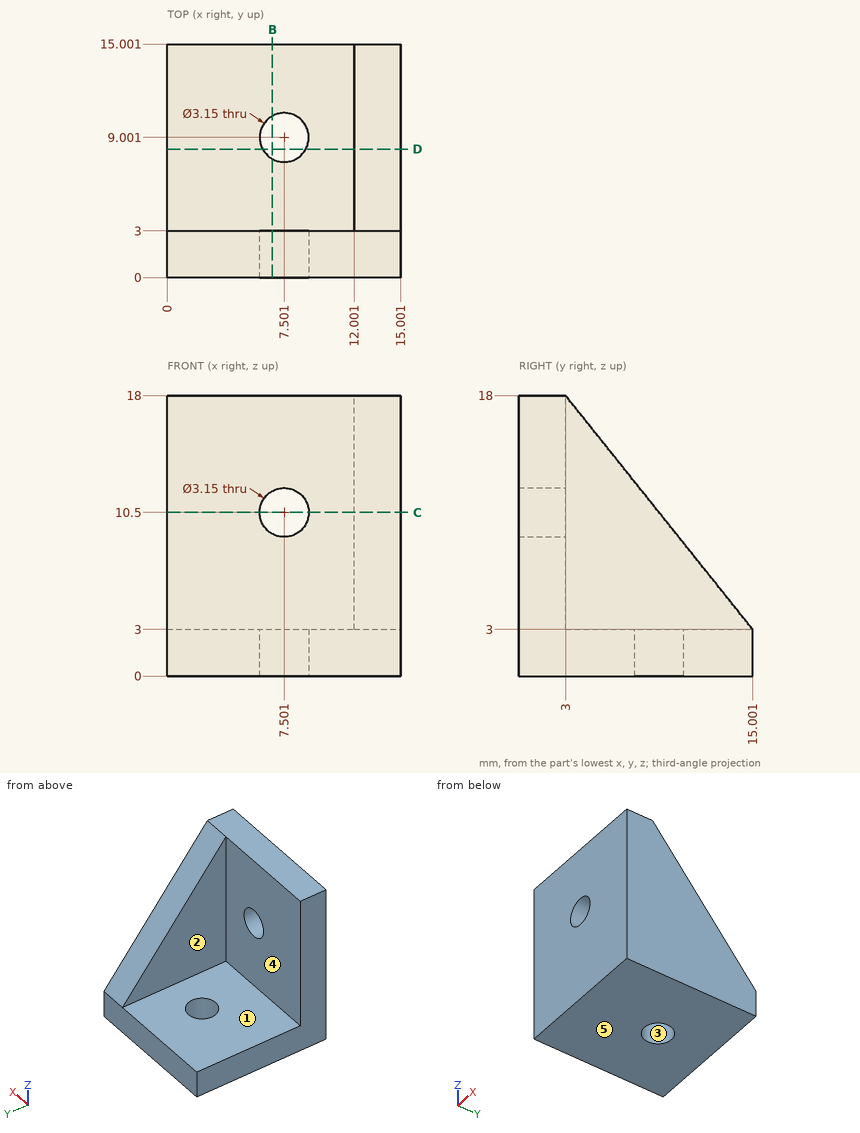
Could you check a few things on this drawing? It's one solid part, dimensions in mm from its lowest x, y, z. A direction names the side the tool comes from. Round coordinates to 2 decimals unless told otherwise and drop trailing zeros. Write each loop counter-clockwise with the first axis right and the second up, starting at its lowest first coordinate (ties: lowest second). Pieces come first, ordered by that corner, then holes. Notation, with made-up numbers: (74, -19.5) -> (102, -19.5) arc R32 ccw to (102, 15.5) -> close; hole circle Ø11 at (67.5, 12). An arc over 180 degrees is marked (long way). Use one line per item in the form item = value. Start each with the question number.
Q1. Imagine slicing it at D-D (y = 8.25). Please give me the cut outline in (x, z) (1 decimal).
Q2. We'd pull the mould along X, two halves only. Please class the marked faces 1, 2 and 3: +X half, -X half, draft (parallel to the pull), parting line (faces both ways), or undercut.
Q3. Which directions (+Z, -Z, +X, -X, +Y, -Y) give clear straight access to the entire face, cutting with the end or side of a thin tool? Please do the marked faces 4 and 5.
Q4. I'm going to push flat-ended pins straight in: P1, Ø3.5, axis at y = 8, z = 12.5, coming from the -X side; P2, Ø2, axis at x = 2.5, z = 16, coming from the +Y side; P3, Ø1.5, axis at x = 4, y = 5, coming from the +Z side. Where does each tip first touch, or does it pass through?
Q5. Imagine slicing it at C-C (z = 10.5). Please give me the cut outline in (x, y) (1 decimal).
Q6. If I drill on probe 1 along X at (y, z) = (1.8, 10.5) (1 decimal); probe 2 along Z at (x, y) = (3.5, 12.5), over which ranges is the centre line in solid material (lowest first)? Write a range as [from, to].
Q7. Imagine slicing it at B-B (x = 6.75). Please give me the cut outline in (y, z) (1 decimal).
Worked out:
q1.outline = (0, 0) -> (6.1, 0) -> (6.1, 3) -> (0, 3) -> close; (8.9, 0) -> (15, 0) -> (15, 11.4) -> (12, 11.4) -> (12, 3) -> (8.9, 3) -> close
q2.face_1 = draft
q2.face_2 = -X half
q2.face_3 = undercut
q3.face_4 = +Z, -X, +Y
q3.face_5 = -Z, +X, -X, +Y, -Y
q4.P1 = 12
q4.P2 = 3
q4.P3 = 3
q5.outline = (0, 0) -> (5.9, 0) -> (5.9, 3) -> (0, 3) -> close; (9.1, 0) -> (15, 0) -> (15, 9) -> (12, 9) -> (12, 3) -> (9.1, 3) -> close
q6.probe_1 = [0, 5.9], [9.1, 15]
q6.probe_2 = [0, 3]
q7.outline = (0, 0) -> (7.6, 0) -> (7.6, 3) -> (3, 3) -> (3, 9.1) -> (0, 9.1) -> close; (0, 11.9) -> (3, 11.9) -> (3, 18) -> (0, 18) -> close; (10.4, 0) -> (15, 0) -> (15, 3) -> (10.4, 3) -> close
